```python
from build123d import *

# Parameters (mm, degrees)
CROQUIS3_R                   = 12.7
SALIENTE_EXTRUIR1_DEPTH      = 50.8
SALIENTE_EXTRUIR1_DEPTH_BACK = 88.9
CROQUIS4_W                   = 31.75
CROQUIS4_H                   = 31.75
SALIENTE_EXTRUIR2_DEPTH      = 38.1
CROQUIS6_W                   = 25.4
CROQUIS6_H                   = 31.75
SALIENTE_EXTRUIR3_DEPTH      = 114.3
CROQUIS8_W                   = 31.75
CROQUIS8_H                   = 31.75
SALIENTE_EXTRUIR4_DEPTH      = 19.05
CROQUIS9_R                   = 6.35
SALIENTE_EXTRUIR5_DEPTH      = 19.05
REDONDEO1_R                  = 6.35
CROQUIS12_W                  = 31.75
CROQUIS12_H                  = 31.75
SALIENTE_EXTRUIR6_DEPTH      = 38.1
CROQUIS13_W                  = 25.4
CROQUIS13_H                  = 31.75
SALIENTE_EXTRUIR7_DEPTH      = 114.3
CROQUIS14_W                  = 31.75
CROQUIS14_H                  = 31.75
SALIENTE_EXTRUIR8_DEPTH      = 19.05
CROQUIS16_R                  = 6.35
SALIENTE_EXTRUIR9_DEPTH      = 19.05
REDONDEO2_R                  = 6.35


with BuildPart() as part:
    # Croquis3 → Saliente-Extruir1 (new body, two sides)
    with BuildSketch(Plane.XY) as saliente_extruir1_sk:
        Circle(CROQUIS3_R)
    extrude(amount=SALIENTE_EXTRUIR1_DEPTH)
    extrude(saliente_extruir1_sk.sketch, amount=-SALIENTE_EXTRUIR1_DEPTH_BACK)

    # Croquis4 → Saliente-Extruir2 (add)
    with BuildSketch(Plane(origin=(0, 0, -88.9), x_dir=(-1, 0, 0), z_dir=(0, 0, -1))):
        Rectangle(CROQUIS4_W, CROQUIS4_H)
    extrude(amount=SALIENTE_EXTRUIR2_DEPTH)

    # Croquis6 → Saliente-Extruir3 (add)
    with BuildSketch(Plane.ZY.offset(15.875)):
        with Locations((-114.3, 0)):
            Rectangle(CROQUIS6_W, CROQUIS6_H)
    extrude(amount=SALIENTE_EXTRUIR3_DEPTH)

    # Croquis8 → Saliente-Extruir4 (add)
    with BuildSketch(Plane(origin=(0, 0, -127), x_dir=(-1, 0, 0), z_dir=(0, 0, -1))):
        with Locations((114.3, 0)):
            Rectangle(CROQUIS8_W, CROQUIS8_H)
    extrude(amount=SALIENTE_EXTRUIR4_DEPTH)

    # Croquis9 → Saliente-Extruir5 (add)
    with BuildSketch(Plane(origin=(0, 0, -146.05), x_dir=(-1, 0, 0), z_dir=(0, 0, -1))):
        with Locations((114.3, 0)):
            Circle(CROQUIS9_R)
    extrude(amount=SALIENTE_EXTRUIR5_DEPTH)

    # Redondeo1
    redondeo1_edges = [part.edges().sort_by_distance(p)[0] for p in [
        (15.875, 0, -127),
        (-41.275, -15.875, -127),
        (-15.875, 15.875, -95.25),
        (-15.875, -15.875, -95.25),
        (-15.875, 0, -101.6),
        (-73.025, -15.875, -101.6),
        (-73.025, 15.875, -101.6),
        (-130.175, -15.875, -123.825),
        (-130.175, 0, -101.6),
        (-130.175, 15.875, -123.825),
        (-41.275, 15.875, -127),
        (-98.425, 0, -127),
        (-98.425, 15.875, -136.525),
        (-98.425, -15.875, -136.525),
        (15.875, 15.875, -107.95),
        (15.875, -15.875, -107.95),
    ]]
    fillet(redondeo1_edges, radius=REDONDEO1_R)

    # Croquis12 → Saliente-Extruir6 (add)
    with BuildSketch(Plane.XY.offset(50.8)):
        Rectangle(CROQUIS12_W, CROQUIS12_H)
    extrude(amount=SALIENTE_EXTRUIR6_DEPTH)

    # Croquis13 → Saliente-Extruir7 (add)
    with BuildSketch(Plane(origin=(15.875, 0, 0), x_dir=(0, 0, -1), z_dir=(1, 0, 0))):
        with Locations((-76.2, 0)):
            Rectangle(CROQUIS13_W, CROQUIS13_H)
    extrude(amount=SALIENTE_EXTRUIR7_DEPTH)

    # Croquis14 → Saliente-Extruir8 (add)
    with BuildSketch(Plane.XY.offset(88.9)):
        with Locations((114.3, 0)):
            Rectangle(CROQUIS14_W, CROQUIS14_H)
    extrude(amount=SALIENTE_EXTRUIR8_DEPTH)

    # Croquis16 → Saliente-Extruir9 (add)
    with BuildSketch(Plane.XY.offset(107.95)):
        with Locations((114.3, 0)):
            Circle(CROQUIS16_R)
    extrude(amount=SALIENTE_EXTRUIR9_DEPTH)

    # Redondeo2
    redondeo2_edges = [part.edges().sort_by_distance(p)[0] for p in [
        (-15.875, 15.875, 69.85),
        (-15.875, -15.875, 69.85),
        (-15.875, 0, 88.9),
        (41.275, -15.875, 88.9),
        (15.875, 15.875, 57.15),
        (15.875, -15.875, 57.15),
        (15.875, 0, 63.5),
        (73.025, -15.875, 63.5),
        (73.025, 15.875, 63.5),
        (130.175, -15.875, 85.725),
        (130.175, 0, 63.5),
        (130.175, 15.875, 85.725),
        (41.275, 15.875, 88.9),
        (98.425, 15.875, 98.425),
        (98.425, -15.875, 98.425),
    ]]
    fillet(redondeo2_edges, radius=REDONDEO2_R)


solid = part.part
```
Geometry check sheet. Reference: the model listing, model coordinates, mm. A direction names the side the tool comes from. Give positions to 0.01 mm unless a question says otherwise; leave off trailing zeros. Loops run counter-clockwise (first coordinate to the right, second up) from the corner with the lowest first, then second, coordinate; pieces in that order, holes last. Notation, with made-up numbers: M 28.5,68 L 50.5,68 A20 ccw 50.5,84 Z; hole C -28,21.5 d5. An arc over 180 degrees is marked long. Write item = value, one per line. Start each with the question number.
1. Section check A-A, the plane x = -54.5. Enter the section's corners in (y, z) (3 decimals), plus the area to 3 significant figures.
2. Draft check along Z on faces 6 (the face through (-7, 11, 50.8)), 7 (the face through (15.875, 0, -105)), 8 (the face through (48.425, -14.064, 86.99)). Enter one of: +Z half, -Z half, draft (parallel to the pull), parting line (faces both ways), or undercut.
3. Thickness scan on probe 1 along Z at (x, y) = (-91.5, 5); probe 2 along Z at (x, y) = (2.5, -8); probe 3 along X at (y, z) = (-2, -135) (3 decimals). Record the ranges inside material, lowest first.
4. Section check B-B, the plane x = 114.3. Enter the section's corners in (y, z) (3 decimals).
5. Go/stop test with flat-tipped pins: P1, Ø15, axis at x = -41.5, y = -1, coming from the -Z side; P2, Ø5.5, axis at x = -83.5, y = -1, coming from the +Z side; P3, Ø14, axis at y = 4.5, z = -140, coming from the +X side. Record where each tip stops, or that it passes through.
6. Tool access check on faces 1 (the face through (-13.97, -14.06, 66.9)), 2 (the face through (-41.986, -14.064, -125.09)), 3 (the face through (-100.24, 13.97, -139.79)), 4 (the face through (46.825, 14.064, 86.99)), 5 (the face through (98.425, 0, 98)). Record the directions out of +Z, -Z, +X, -X, +Y, -Y that give a thin tool (end or side, any length) a straight path to the whole face; none if there is none.
7. Section check C-C, the plane x = 0. Enter the section's corners in (y, z) (3 decimals), plus the area to 3 significant figures.
Values follow:
q1.outline = M -15.875,-120.65 A6.35 ccw -9.525,-127 L 9.525,-127 A6.35 ccw 15.875,-120.65 L 15.875,-107.95 A6.35 ccw 9.525,-101.6 L -9.525,-101.6 A6.35 ccw -15.875,-107.95 Z
q1.area = 772 mm^2
q2.face_6 = undercut
q2.face_7 = draft
q2.face_8 = +Z half
q3.probe_1 = -127 to -101.6
q3.probe_2 = -127 to 88.9
q3.probe_3 = -130.175 to -98.425
q4.outline = M -15.875,69.85 A6.35 ccw -9.525,63.5 L 9.525,63.5 A6.35 ccw 15.875,69.85 L 15.875,107.95 L 6.35,107.95 L 6.35,127 L -6.35,127 L -6.35,107.95 L -15.875,107.95 Z
q5.P1 = -127
q5.P2 = -101.6
q5.P3 = -98.42
q6.face_1 = +Z, -X, -Y
q6.face_2 = -Z, +X, -Y
q6.face_3 = -Z, +X, +Y
q6.face_4 = +Z, -X, +Y
q6.face_5 = +Z, -X, +Y, -Y
q7.outline = M -15.875,-120.65 A6.35 ccw -9.525,-127 L 9.525,-127 A6.35 ccw 15.875,-120.65 L 15.875,-88.9 L 12.7,-88.9 L 12.7,50.8 L 15.875,50.8 L 15.875,82.55 A6.35 ccw 9.525,88.9 L -9.525,88.9 A6.35 ccw -15.875,82.55 L -15.875,50.8 L -12.7,50.8 L -12.7,-88.9 L -15.875,-88.9 Z
q7.area = 5,930 mm^2
